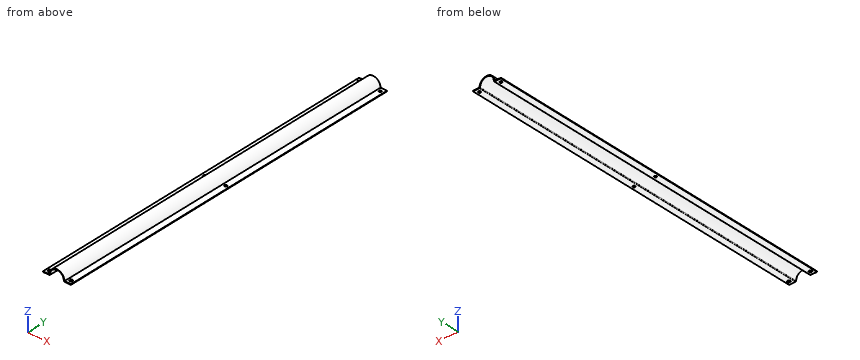
from build123d import *

# Parameters (mm, degrees)
F1_DEPTH = 559.5
F2_R     = 1.9
F2_R_2   = 2.2432813823
F3_DEPTH = 1


# Not quite as in the source:
# - a pattern or mirror of a feature is missing from the dataset's text; its kind, count and spacing are read off the source's solid
# - a feature names something its author has since deleted; it is built from what else it names


with BuildPart() as f1:
    # F0 (on Front) → F1 (new body)
    with BuildSketch(Plane.XZ):
        with BuildLine():
            Line((-21.5, 0), (-21.5, -1))
            Line((-21.5, -1), (-11.5475115549, -1))
            ThreePointArc((-11.5475115549, -1), (-10.8404047737, -0.7071067812), (-10.5475115549, 0))
            ThreePointArc((-10.5475115549, 0), (0, 10.5475115549), (10.5475115549, 0))
            ThreePointArc((10.5475115549, 0), (10.8404047737, -0.7071067812), (11.5475115549, -1))
            Line((11.5475115549, -1), (21.5, -1))
            Line((21.5, -1), (21.5, 0))
            Line((21.5, 0), (11.5, 0))
            ThreePointArc((11.5, 0), (0, 11.5), (-11.5, 0))
            Line((-11.5, 0), (-21.5, 0))
        make_face()
    extrude(amount=F1_DEPTH)

    # F2 (on face) → F3 (cut, through all)
    with BuildSketch(Plane.XY):
        with Locations((16.5, -279.50005)):
            Circle(F2_R)
        with Locations((16.5, -6)):
            Circle(F2_R)
        with Locations((16.5236079696, -553.5000464449)):
            Circle(F2_R_2)
    f3 = extrude(amount=-F3_DEPTH, mode=Mode.SUBTRACT)

    # F3_copies: F3 across plane
    add(f3.mirror(Plane(origin=(0, 0, 0), x_dir=(0, 0, -1), z_dir=(-1, 0, 0))), mode=Mode.SUBTRACT)


solid = f1.part
For this review, take the finished solid that the model builds, in its own axes (mm). Round coordinates to 2 decimals unless told otherwise and drop trailing zeros. Loops run counter-clockwise (first coordinate to the right, second up) from the corner with the lowest first, then second, coordinate; pieces in that order, holes last. Notation, with made-up numbers: (23, -6.5) - (28, -6.5) arc R19 ccw to (28, 5.5) - close; hole circle Ø4 at (78.5, 81). An arc over 180 degrees is marked (long way). One line per question, with ' | ' between items.
Q1. Take a section at B-B (y = -407.5). Give the boundary of the cut face in (x, z).
Taken from the geometry:
outline: (-21.5, -1) - (-11.55, -1) arc R1 ccw to (-10.55, 0) arc R10.55 cw to (10.55, 0) arc R1 ccw to (11.55, -1) - (21.5, -1) - (21.5, 0) - (11.5, 0) arc R11.5 ccw to (-11.5, 0) - (-21.5, 0) - close
Q2. For line 1 along Y through (x, z) = (16, -0.5); line 2 along Y through (x, z) = (16.5, -0.3); line 3 along X through (y, z) = (-523.5, 0.5), list the stretches that pass through material, from the lowest coordinate up. Write a range as [from, to].
Taken from the geometry:
line 1: y = [-559.5, -555.68], [-551.32, -281.33], [-277.67, -7.83], [-4.17, 0] | line 2: y = [-559.5, -555.74], [-551.26, -281.4], [-277.6, -7.9], [-4.1, 0] | line 3: x = [-11.49, -10.54], [10.54, 11.49]
Q3. For pin 1 (4.5 mm diameter, centred on x = -16.5, y = -6, fed in from +Z); pin 2 (6 mm diameter, centred on x = -10.5, z = 5.5, fed in from +Y); pin 3 (4 mm diameter, centred on y = -95, z = 7, fed in from -X); pin 4 (10 mm diameter, centred on x = -0.5, y = -410, fed in from -Z), all flat-tipped, find the tip position at first contact; note any pin that passes through.
Taken from the geometry:
pin 1: stops at z = 0 | pin 2: stops at y = 0 | pin 3: stops at x = -10.36 | pin 4: stops at z = 9
Q4. Take a section at A-A (z = 4.75). Give the boundary of the cut face in (x, y), and give its area (3 significant figures).
Taken from the geometry:
outline: (-10.47, -559.5) - (-9.42, -559.5) - (-9.42, 0) - (-10.47, 0) - close; (9.42, -559.5) - (10.47, -559.5) - (10.47, 0) - (9.42, 0) - close | area: 1,180 mm²
Q5. Take a section at C-C (x = 0). Give the boundary of the cut face in (y, z).
Taken from the geometry:
outline: (-559.5, 10.55) - (0, 10.55) - (0, 11.5) - (-559.5, 11.5) - close
